from build123d import *

# Parameters (mm, degrees)
SKETCH1_R           = 6.25
BOSS_EXTRUDE1_DEPTH = 1
SKETCH2_R           = 5.5
BOSS_EXTRUDE2_DEPTH = 3
SKETCH3_R           = 3
BOSS_EXTRUDE3_DEPTH = 1
SKETCH4_R           = 2
BOSS_EXTRUDE4_DEPTH = 5
CHAMFER1_SIZE       = 0.25
CHAMFER2_SIZE       = 0.25


with BuildPart() as part:
    # Sketch1 → Boss-Extrude1 (new body)
    with BuildSketch(Plane(origin=(0, 0, 0), x_dir=(1, 0, 0), z_dir=(0, 1, 0))):
        with Locations(Location((0, 0, 0), (0, 0, 270))):
            Circle(SKETCH1_R)
    extrude(amount=BOSS_EXTRUDE1_DEPTH)

    # Sketch2 → Boss-Extrude2 (add)
    with BuildSketch(Plane.XZ):
        with Locations(Location((0, 0, 0), (0, 0, 270))):
            Circle(SKETCH2_R)
    extrude(amount=BOSS_EXTRUDE2_DEPTH)

    # Sketch3 → Boss-Extrude3 (add)
    with BuildSketch(Plane(origin=(0, 1, 0), x_dir=(1, 0, 0), z_dir=(0, 1, 0))):
        with Locations(Location((0, 0, 0), (0, 0, 270))):
            Circle(SKETCH3_R)
    extrude(amount=BOSS_EXTRUDE3_DEPTH)

    # Sketch4 → Boss-Extrude4 (add)
    with BuildSketch(Plane(origin=(0, 2, 0), x_dir=(1, 0, 0), z_dir=(0, 1, 0))):
        with Locations(Location((0, 0, 0), (0, 0, 270))):
            Circle(SKETCH4_R)
    extrude(amount=BOSS_EXTRUDE4_DEPTH)

    # Chamfer1
    chamfer1_edges = [part.edges().sort_by_distance(p)[0] for p in [
        (0, 0, -6.25),
        (0, 1, -6.25),
        (0, -3, 5.5),
    ]]
    chamfer(chamfer1_edges, length=CHAMFER1_SIZE)

    # Chamfer2
    chamfer2_edges = [part.edges().sort_by_distance(p)[0] for p in [
        (0, 2, -3),
    ]]
    chamfer(chamfer2_edges, length=CHAMFER2_SIZE)


solid = part.part
Could you check a few things on this model? Use its own coordinates, in mm. A direction names the side the tool comes from. Round coordinates to 2 decimals unless told otherwise and drop trailing zeros. Order: outer loops, then holes, each group sorted by start corner. A loop starts at its lowest first (then second) coordinate and runs counter-clockwise, first axis right, second up. Notation, with made-up numbers: M -32,-40 L 24,-40 A25 cw 24,-27 Z; hole C 51,69 d1. An arc over 180 degrees is marked long. One line per item, written item: value.
(1) Imagine slicing it at B-B (x = 0). Write out the boundary of the cut face in (y, z), and give its area (4 significant figures).
Ans:
outline: M -3,-5.25 L -2.75,-5.5 L 0,-5.5 L 0,-6 L 0.25,-6.25 L 0.75,-6.25 L 1,-6 L 1,-3 L 1.75,-3 L 2,-2.75 L 2,-2 L 7,-2 L 7,2 L 2,2 L 2,2.75 L 1.75,3 L 1,3 L 1,6 L 0.75,6.25 L 0.25,6.25 L 0,6 L 0,5.5 L -2.75,5.5 L -3,5.25 Z
area: 71.25 mm^2
(2) Imagine slicing it at D-D (y = 0.5). Write out the boundary of the cut face in (x, z), and give its area (3 significant figures).
Ans:
outline: C 0,0 d12.5
area: 123 mm^2
(3) Imagine slicing it at A-A (z = 0). Write out the boundary of the cut face in (x, y), and give its area (4 significant figures).
Ans:
outline: M -6.25,0.25 L -6,0 L -5.5,0 L -5.5,-2.75 L -5.25,-3 L 5.25,-3 L 5.5,-2.75 L 5.5,0 L 6,0 L 6.25,0.25 L 6.25,0.75 L 6,1 L 3,1 L 3,1.75 L 2.75,2 L 2,2 L 2,7 L -2,7 L -2,2 L -2.75,2 L -3,1.75 L -3,1 L -6,1 L -6.25,0.75 Z
area: 71.25 mm^2
(4) I'm going to push flat-ended pins straight in: P1, Ø5, axis at y = 6, z = 4, coming from the +X side; P2, Ø2, axis at x = -2, z = 4, coming from the +Y side; P3, Ø1, axis at y = 2, z = 2.5, coming from the +X side. Where does each tip first touch, or does it pass through?
Ans:
P1: stops at x = 1.32
P2: stops at y = 1
P3: stops at x = 2.17
(5) Which directions (+Z, -Z, +X, -X, +Y, -Y) give clear straight access to the entire face, cutting with the end or side of a thin tool? Please do faces 1 (the cylindrical face through (0.9, 1.37, 2.86)), 2 (the flat face through (0, -3, 0)), 3 (the cylindrical face through (-5.37, -1.36, 1.19)).
Ans:
face 1: +Y
face 2: +Z, -Z, +X, -X, -Y
face 3: -Y
(6) I need wall thicknesses on line 1 along Y through (x, z) = (3.25, 5); line 2 along Y through (x, z) = (2.75, -2); line 3 along X through (y, z) = (-1.75, -1.5). Which ranges of each line are inside material? Lowest first, please. Write a range as from..to.
Ans:
line 1: y = 0..1
line 2: y = -3..1
line 3: x = -5.29..5.29
(7) Imagine slicing it at C-C (y = 6.75). Write out the boundary of the cut face in (x, z).
Ans:
outline: C 0,0 d4
